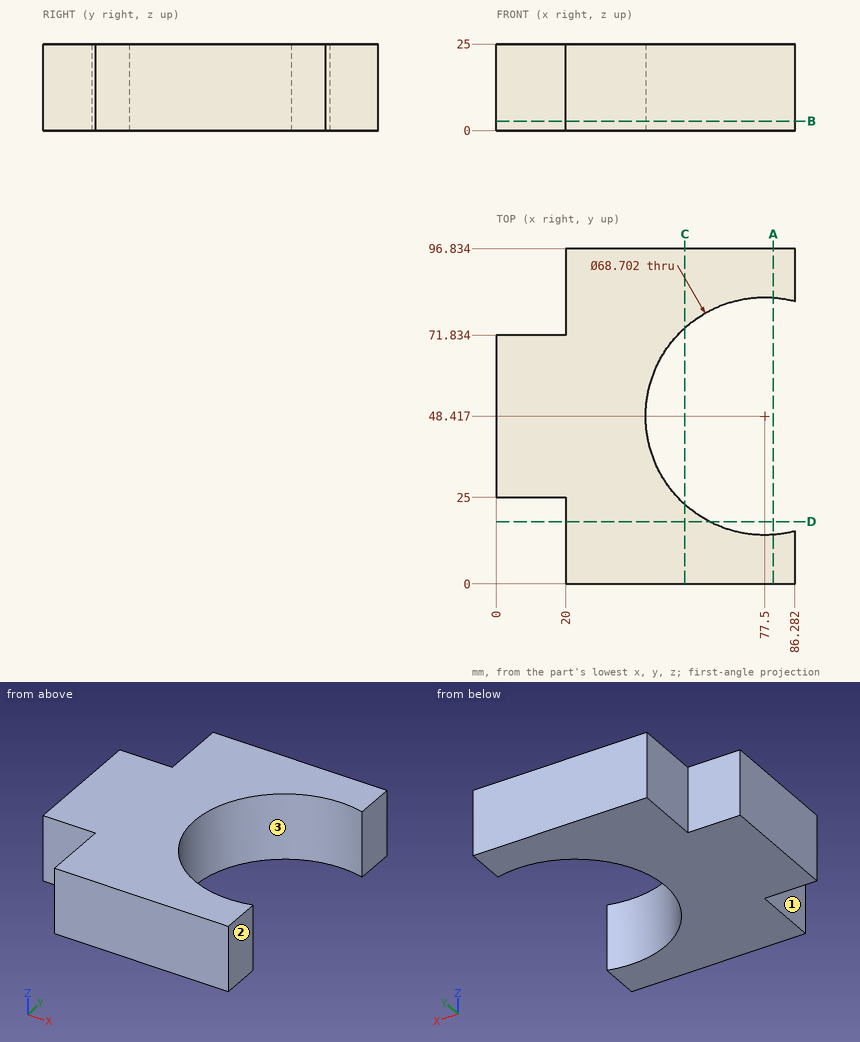
Source: three-view drawing plus pictorial views. Frame: mm from the lowest corner of the part. Give positions to 0.01 mm unless a question says otherwise; leave off trailing zeros. Order: outer loops, then holes, each group sorted by start corner. A loop starts at its lowest first (then second) coordinate and runs counter-clockwise, first axis right, second up. Notation, with made-up numbers: M 13.5,-33.5 L 32.5,-33.5 A12 ccw 32.5,-23.5 Z; hole C 87.25,25 d2. An arc over 180 degrees is marked long. One line per question, with ' | ' between items.
1) Contact query for flat-ended pins moving along their axis: P1, Ø12.5, axis at y = 17.5, z = 8, coming from the -X side; P2, Ø6, axis at x = 11, z = 17, coming from the +Y side; P3, Ø10, axis at y = 60, z = 9, coming from the +X side. Output: stop coordinate, or through.
Filled in:
P1: stops at x = 20 | P2: stops at y = 71.83 | P3: stops at x = 47.42
2) Section D-D on y = 18. Output: boundary loops of the cut face in (x, z), and give its area (3 significant figures).
Filled in:
outline: M 20,0 L 61.54,0 L 61.54,25 L 20,25 Z | area: 1,040 mm2
3) Draft query along X for the marked faces 1, 2 and 3. Return one class per face: pulls with the +X half, pulls with the -X half, needs draft (parallel to the pull), parting line crosses it, or undercut.
Filled in:
face 1: pulls with the -X half | face 2: pulls with the +X half | face 3: undercut
4) Ray query, L1, parallel to X at y = 6, z = 18.75; L2, parallel to Y at x = 68, z = 7.75 (1 decimal); L3, parallel to X at y = 47.5, z = 17.5. Return the intervals inside material, ascending.
Filled in:
L1: x = 20 to 86.28 | L2: y = 0 to 15.4, 81.4 to 96.8 | L3: x = 0 to 43.16
5) Section A-A on x = 80. Output: boundary loops of the cut face in (y, z), and give its area (3 significant figures).
Filled in:
outline: M 0,0 L 14.16,0 L 14.16,25 L 0,25 Z; M 82.68,0 L 96.83,0 L 96.83,25 L 82.68,25 Z | area: 708 mm2
6) Section B-B on z = 2.75. Output: boundary loops of the cut face in (x, y).
Filled in:
outline: M 0,25 L 20,25 L 20,0 L 86.28,0 L 86.28,15.21 A34.35 cw long 86.28,81.63 L 86.28,96.83 L 20,96.83 L 20,71.83 L 0,71.83 Z
7) Section C-C on x = 54.5. Output: boundary loops of the cut face in (y, z).
Filled in:
outline: M 0,0 L 22.9,0 L 22.9,25 L 0,25 Z; M 73.93,0 L 96.83,0 L 96.83,25 L 73.93,25 Z
